CAD build for the part. Positions are in the model's coordinates, mm. Round coordinates to 2 decimals unless told otherwise and drop trailing zeros. Write each loop counter-clockwise with the first axis right and the second up, starting at its lowest first coordinate (ties: lowest second). Pieces come first, ordered by that corner, then holes. Notation, with made-up numbers: (-27.5, 63.5) - (3.5, 63.5) arc R12 cw to (3.5, 72.5) - close; hole circle Ø2 at (-3, 0). An arc over 180 degrees is marked (long way). Put each result on its own line as item: value. Start each with the question number.
Item 1: Pin check, flat tip, straight feed: pin 1 Ø2 at (x, y) = (11.5, -1.5) entering from -Z. Stop position of the tip, or through.
Item 2: Cut at A-A (y = 2). Give the cut face in (x, z), and give its area (3 significant figures).
Item 3: Drill centre lines: line 1 (Z direction, x = -8.5, y = 1.3); line 2 (Z direction, x = -15, y = -1.8); line 3 (X direction, y = 1.4, z = 46). Where is each one in solid material? Low to high. Write a range as from..to.
```python
from build123d import *

# Parameters (mm, degrees)
BOSS_EXTRUDE1_DEPTH = 50.000000076
FILLET1_R           = 1.27


with BuildPart() as part:
    # Sketch2 → Boss-Extrude1 (new body)
    with BuildSketch(Plane.XY):
        with BuildLine():
            Line((-15.73, -2.5), (15.73, -2.5))
            ThreePointArc((15.73, -2.5), (16.628025612, -2.128025612), (17, -1.23))
            Line((17, -1.23), (17, 1.23))
            ThreePointArc((17, 1.23), (16.628025612, 2.128025612), (15.73, 2.5))
            Line((15.73, 2.5), (-15.73, 2.5))
            ThreePointArc((-15.73, 2.5), (-16.628025612, 2.128025612), (-17, 1.23))
            Line((-17, 1.23), (-17, -1.23))
            ThreePointArc((-17, -1.23), (-16.628025612, -2.128025612), (-15.73, -2.5))
        make_face()
    extrude(amount=BOSS_EXTRUDE1_DEPTH)

    # Fillet1
    fillet1_edges = [part.edges().sort_by_distance(p)[0] for p in [
        (17, 0, 0),
        (16.628025612, -2.128025612, 0),
        (0, -2.5, 0),
        (-16.628025612, -2.128025612, 0),
        (16.628025612, -2.128025612, 50.000000076),
        (17, 0, 50.000000076),
        (16.628025612, 2.128025612, 50.000000076),
        (0, 2.5, 50.000000076),
        (-16.628025612, 2.128025612, 50.000000076),
        (-17, 0, 50.000000076),
        (-16.628025612, -2.128025612, 50.000000076),
        (-17, 0, 0),
        (0, -2.5, 50.000000076),
        (-16.628025612, 2.128025612, 0),
        (0, 2.5, 0),
        (16.628025612, 2.128025612, 0),
    ]]
    fillet(fillet1_edges, radius=FILLET1_R)


solid = part.part
```
Output values:
1. pin 1: z = 0
2. outline: (-16.74, 1.27) arc R1.01 ccw to (-15.73, 0.26) - (15.73, 0.26) arc R1.01 ccw to (16.74, 1.27) - (16.74, 48.73) arc R1.01 ccw to (15.73, 49.74) - (-15.73, 49.74) arc R1.01 ccw to (-16.74, 48.73) - close
2. area: 1,660 mm2
3. line 1: 0..50
3. line 2: 0.14..49.86
3. line 3: -16.99..16.99
